Study the drawing (mm; zero at the part's minimum x, y, z) and answer. Coordinates: 2 decimals unless noted, no trailing zeros. Order: outer loops, then holes, each group sorted by start corner. A loop starts at its lowest first (then second) coordinate and runs counter-clockwise, first axis right, second up. Notation, with made-up numbers: (30, 39) -> (66, 39) arc R24 ccw to (66, 65) -> close; hole circle Ø1 at (78, -17.5). An arc over 180 degrees is marked (long way). Answer as CSV lines item,"result". Start each with the question number.
Item 1: This flat-tipped pin is pushed along its axis until it touches: pin 1 Ø6 at (x, y) = (13.5, 1.5) entering from -Z. Where does it stop, or does it pass through?
Item 2: Straight lines are drawn through the part: L1, parallel to Z at x = 27, y = 10.25; L2, parallel to Z at x = 32.5, y = 11.25; L3, parallel to Y at x = 10.5, z = 2.5. For each, find the intervals that lie inside material, in ascending order.
Item 3: Section A-A (z = 34.5) is taken. Write down the section's boundary in (x, y), then the cut area to 3 significant figures.
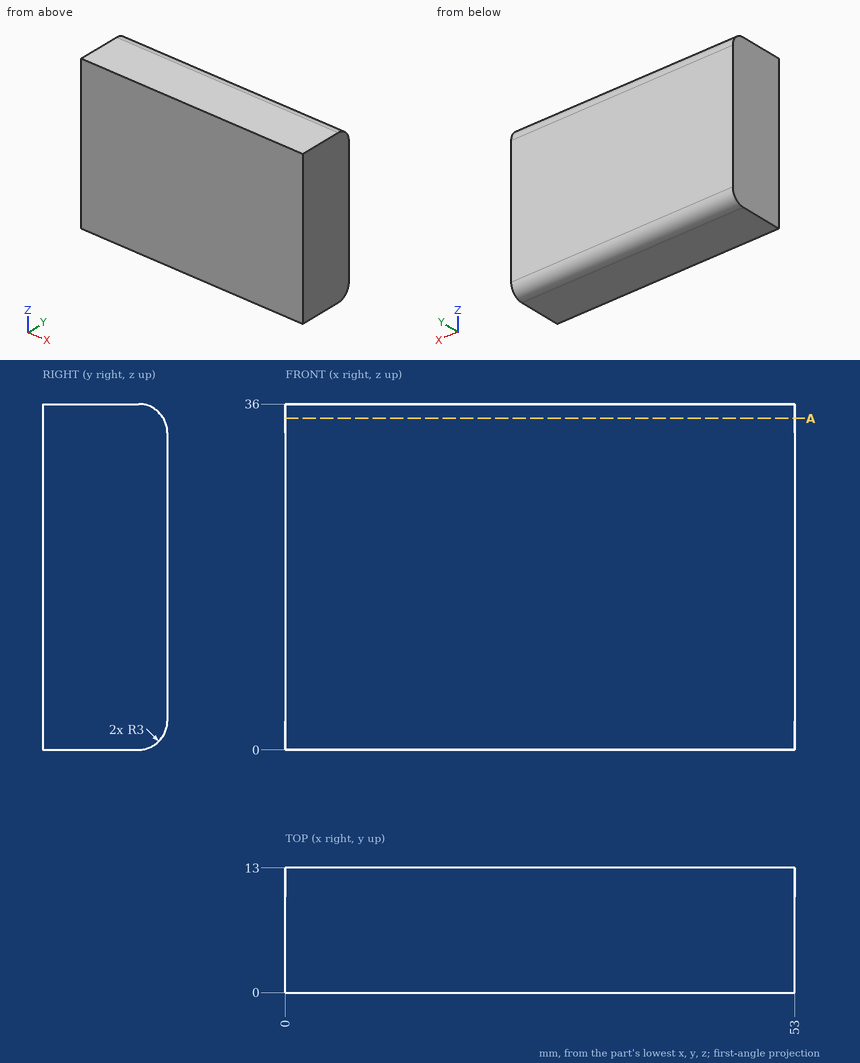
Checked values:
1,pin 1,"stops at z = 0"
2,L1,"z = 0.01 to 35.99"
2,L2,"z = 0.27 to 35.73"
2,L3,"y = 0 to 12.96"
3,outline,"(0, 0) -> (53, 0) -> (53, 12.6) -> (0, 12.6) -> close"
3,area,"668 mm^2"
